```python
from build123d import *

# Parameters (mm, degrees)
PAD_DEPTH    = 60
SKETCH001_W  = 46
SKETCH001_H  = 60
SKETCH001_R  = 2.55
PAD001_DEPTH = 4
SKETCH002_R  = 3
HOLE_DEPTH   = 31.001


with BuildPart() as part:
    # Sketch → Pad (new body)
    with BuildSketch(Plane.XY):
        Polygon((-8, 0), (8, 0), (8, 343), (4.05, 343), (4.05, 330), (-4.05, 330), (-4.05, 343), (-8, 343), align=None)
    extrude(amount=PAD_DEPTH)

    # Sketch001 (on Face3 of Pad) → Pad001 (join)
    with BuildSketch(Plane.XZ):
        with Locations((0, 30)):
            Rectangle(SKETCH001_W, SKETCH001_H)
        with Locations((-14.5, 10)):
            Circle(SKETCH001_R, mode=Mode.SUBTRACT)
        with Locations((-14.5, 50)):
            Circle(SKETCH001_R, mode=Mode.SUBTRACT)
        with Locations((-14.5, 30)):
            Circle(SKETCH001_R, mode=Mode.SUBTRACT)
        with Locations((14.5, 50)):
            Circle(SKETCH001_R, mode=Mode.SUBTRACT)
        with Locations((14.5, 30)):
            Circle(SKETCH001_R, mode=Mode.SUBTRACT)
        with Locations((14.5, 10)):
            Circle(SKETCH001_R, mode=Mode.SUBTRACT)
    extrude(amount=-PAD001_DEPTH)

    # Sketch002 (on Face3 of Pad001) → Hole (cut, through all)
    with BuildSketch(Plane(origin=(-8, 0, 0), x_dir=(0, -1, 0), z_dir=(-1, 0, 0))):
        with Locations((-336.5, 50)):
            Circle(SKETCH002_R)
        with Locations((-336.5, 10)):
            Circle(SKETCH002_R)
        with Locations((-336.5, 30)):
            Circle(SKETCH002_R)
    extrude(amount=-HOLE_DEPTH, mode=Mode.SUBTRACT)


solid = part.part
```
Source: CAD feature listing. Evaluate the final solid. Frame: model axes, mm. A direction names the side the tool comes from. Round coordinates to 2 decimals unless told otherwise and drop trailing zeros. Loops run counter-clockwise (first coordinate to the right, second up) from the corner with the lowest first, then second, coordinate; pieces in that order, holes last.
1. Mould query, pull axis Y, two halves, no side actions, for faces 6 (the cylindrical face through (6, 333.73, 28.85)), 7 (the flat face through (0, 330, 30)), 8 (the flat face through (0, 158, 60)). Classes: released by +Y, released by -Y, zero draft, split by the parting line, or undercut.
2. Section query B-B on z = 40.5. Output: boundary loops of the cut face in (x, y), and give its area (3 significant figures).
3. Access query for faces 1 (the flat face through (-4.05, 332, 30)), 2 (the flat face through (19, 4, 30)), 3 (the flat face through (0, 0, 30)), 4 (the flat face through (-17.3, 4, 30.4)), 5 (the cylindrical face through (6, 333.64, 50.9)). Directions: +Z, -Z, +X, -X, +Y, -Y. A direction counts if a zero-diameter tool reaches every point of the face in a straight line with its end or side. Return the directions, or none.
4. Contact query for flat-ended pins moving along their axis: pin 1 (3 mm diameter, centred on y = 40, z = 28, fed in from -X); pin 2 (6 mm diameter, centred on x = -14.5, z = 50, fed in from +Y); pin 3 (10 mm diameter, centred on y = 55.5, z = 14, fed in from +X). Output: stop coordinate, or through.
5. Section query A-A on y = 336.5. Give the number of separate pieces and of enclosed holes in the cut face, and give its area (3 significant figures).
6. Ray query, L1, parallel to Z at x = -14, y = 2; L2, parallel to Y at x = -14, z = 33; L3, parallel to X at y = 322, z = 16. Return the intervals inside material, ascending.
Answers below:
1. face 6: undercut
1. face 7: released by +Y
1. face 8: zero draft
2. outline: (-23, 0) - (23, 0) - (23, 4) - (8, 4) - (8, 343) - (4.05, 343) - (4.05, 330) - (-4.05, 330) - (-4.05, 343) - (-8, 343) - (-8, 4) - (-23, 4) - close
2. area: 5,500 mm2
3. face 1: +Z, -Z, +Y
3. face 2: +Z, -Z, +X, +Y
3. face 3: +Z, -Z, +X, -X, -Y
3. face 4: +Z, -Z, -X, +Y
3. face 5: +X, -X
4. pin 1: stops at x = -8
4. pin 2: stops at y = 4
4. pin 3: stops at x = 8
5. separate pieces: 8
5. enclosed holes: 0
5. area: 332 mm2
6. L1: z = 0 to 7.5, 12.5 to 27.5, 32.5 to 47.5, 52.5 to 60
6. L2: y = 0 to 4
6. L3: x = -8 to 8
